Could you check a few things on this model? Use its own coordinates, in mm. Face numbers are marked on the shaded views. A direction names the side the tool comes from. Give positions to 0.01 mm unless a question says otherwise; leave off trailing zeros. Write each loop counter-clockwise with the first axis right and the second up, starting at its lowest first coordinate (ties: lowest second). Pieces come first, ordered by that corner, then holes. Notation, with made-up numbers: M 70.5,27 L 88.5,27 A12 cw 88.5,45 Z; hole C 30,-0.75 d1. An arc over 180 degrees is marked long. One line per item, written item: value.
```python
from build123d import *

# Parameters (mm, degrees)
SKETCH1_R           = 1.4224
BOSS_EXTRUDE1_DEPTH = 12.7
SKETCH2_R           = 2.7051
BOSS_EXTRUDE2_DEPTH = 1.4986
FILLET1_R           = 1.016
CUT_EXTRUDE1_DEPTH  = 2.38125


with BuildPart() as part:
    # Sketch1 → Boss-Extrude1 (new body)
    with BuildSketch(Plane(origin=(0, 0, 0), x_dir=(1, 0, 0), z_dir=(0, 1, 0))):
        Circle(SKETCH1_R)
    extrude(amount=BOSS_EXTRUDE1_DEPTH)

    # Sketch2 → Boss-Extrude2 (add)
    with BuildSketch(Plane(origin=(0, 12.7, 0), x_dir=(1, 0, 0), z_dir=(0, 1, 0))):
        Circle(SKETCH2_R)
    extrude(amount=BOSS_EXTRUDE2_DEPTH)

    # Fillet1
    fillet1_edges = [part.edges().sort_by_distance(p)[0] for p in [
        (-2.7051, 14.1986, 0),
    ]]
    fillet(fillet1_edges, radius=FILLET1_R)

    # Sketch3 → Cut-Extrude1 (cut)
    with BuildSketch(Plane(origin=(0, 14.1986, 0), x_dir=(1, 0, 0), z_dir=(0, 1, 0))):
        Polygon((0, 0.916543552), (-0.79375, 0.458271776), (-0.79375, -0.458271776), (0, -0.916543552), (0.79375, -0.458271776), (0.79375, 0.458271776), align=None)
    extrude(amount=-CUT_EXTRUDE1_DEPTH, mode=Mode.SUBTRACT)


solid = part.part
```
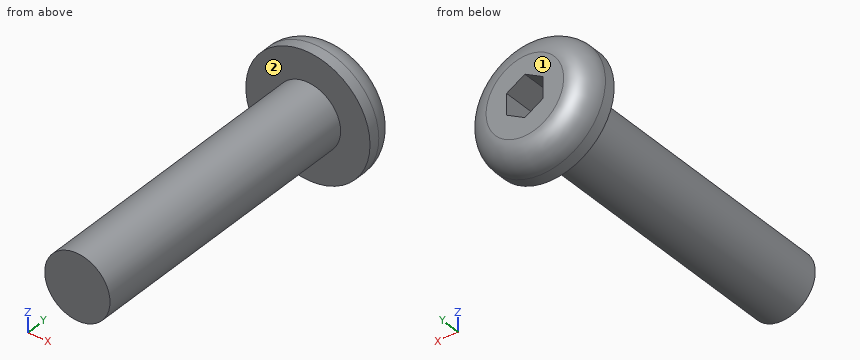
1) On a 3-axis mill with a long thin cutter (end or side, diameter ignored), from which of +Z, -Z, +X, -X, +Y, -Y can I reach the whole of each face in a straight line? I mean the marked faces 1 and 2. Say none if no direction works.
Outcome:
face 1: +Z, -Z, +X, -X, +Y
face 2: -Y
2) If we section it at C-C, the plane y = 4.75: Write out the boundary of the cut face in (x, z).
Outcome:
outline: C 0,0 d2.84
3) I'm going to push flat-ended pins straight in: pin 1 (1 mm diameter, centred on x = 0, y = 9, fed in from +Z); pin 2 (1.5 mm diameter, centred on x = 0.5, y = 10, fed in from -Z). Where does each tip first touch, or does it pass through?
Outcome:
pin 1: stops at z = 1.42
pin 2: stops at z = -1.42
4) If we section it at B-B, the plane z = 0: Write out the boundary of the cut face in (x, y), then the cut area to 3 significant figures.
Outcome:
outline: M -2.71,12.7 L -1.42,12.7 L -1.42,0 L 1.42,0 L 1.42,12.7 L 2.71,12.7 L 2.71,13.18 A1.02 ccw 1.69,14.2 L 0.79,14.2 L 0.79,11.82 L -0.79,11.82 L -0.79,14.2 L -1.69,14.2 A1.02 ccw -2.71,13.18 Z
area: 40.0 mm^2
5) Please list where these lines run through material, in increasing order: L1, parallel to Y at x = 0.4, z = 0.6; L2, parallel to Z at x = -0.1, y = 3; L3, parallel to Y at x = -1.3, z = -0.7. Write a range as from..to.
Outcome:
L1: y = 0..11.82
L2: z = -1.42..1.42
L3: y = 12.7..14.2
6) If we section it at A-A, the plane y = 12.25: Write out the boundary of the cut face in (x, z), then the cut area to 3 significant figures.
Outcome:
outline: C 0,0 d2.84; hole M -0.79,-0.46 L 0,-0.92 L 0.79,-0.46 L 0.79,0.46 L 0,0.92 L -0.79,0.46 Z
area: 4.17 mm^2
